Geometry check sheet. Reference: the model listing, model coordinates, mm. A direction names the side the tool comes from. Round coordinates to 2 decimals unless told otherwise and drop trailing zeros. Write each loop counter-clockwise with the first axis right and the second up, starting at its lowest first coordinate (ties: lowest second). Pieces come first, ordered by that corner, then holes. Notation, with made-up numbers: (31, 6.5) -> (78, 6.5) arc R34 ccw to (78, 45.5) -> close; hole circle Ø8 at (-3, 52). An arc over 180 degrees is marked (long way). Return JSON: item names as keys, results as strings. Group by question number.
from build123d import *

# Parameters (mm, degrees)
SKETCH1_W           = 19.05
SKETCH1_H           = 19.05
BOSS_EXTRUDE1_DEPTH = 5.08
SKETCH2_R           = 8.255
BOSS_EXTRUDE2_DEPTH = 15.24
SKETCH3_R           = 6.35
CUT_EXTRUDE1_DEPTH  = 25.379369352
FILLET1_R           = 2.54


with BuildPart() as part:
    # Sketch1 → Boss-Extrude1 (new body)
    with BuildSketch(Plane.XY):
        Rectangle(SKETCH1_W, SKETCH1_H)
    extrude(amount=-BOSS_EXTRUDE1_DEPTH)

    # Sketch2 → Boss-Extrude2 (add)
    with BuildSketch(Plane(origin=(0, 0, -5.08), x_dir=(-1, 0, 0), z_dir=(0, 0, -1))):
        with Locations(Location((0, 0, 0), (0, 0, 180))):
            Circle(SKETCH2_R)
    extrude(amount=BOSS_EXTRUDE2_DEPTH)

    # Sketch3 → Cut-Extrude1 (cut, through all)
    with BuildSketch(Plane.XY):
        Circle(SKETCH3_R)
    extrude(amount=-CUT_EXTRUDE1_DEPTH, mode=Mode.SUBTRACT)

    # Fillet1
    fillet1_edges = [part.edges().sort_by_distance(p)[0] for p in [
        (9.525, -9.525, -2.54),
        (-9.525, -9.525, -2.54),
        (-9.525, 9.525, -2.54),
        (9.525, 9.525, -2.54),
    ]]
    fillet(fillet1_edges, radius=FILLET1_R)


solid = part.part
1) Material ranges on probe 1 along Y at (x, z) = (0, -12.75) (3 decimals); probe 2 along X at (y, z) = (-0.25, -5) (3 decimals); probe 3 along Z at (x, y) = (-4.75, -8.5), recorded low to high. Write a range as [from, to].
2) Mould release check, pull along X, two halves, no side actions. Record for faces 1 (the face through (-8.8, -8.76, -2.58)), 2 (the face through (9.525, 0, -3)), 3 (the face through (-1.38, -6.2, -10.02)), 4 (the face through (0, -9.525, -3)): +X half, -X half, draft (parallel to the pull), parting line (faces both ways), or undercut.
3) Tool access check on faces 5 (the face through (0, 9.525, -3)), 6 (the face through (7.874, -2.48, -12.593)). Record the directions out of +Z, -Z, +X, -X, +Y, -Y that give a thin tool (end or side, any length) a straight path to the whole face; none if there is none.
4) Sectioned sample at C-C on z = -2.75. Enter the section's corners in (x, y) (3 decimals).
5) Sectioned sample at A-A on y = 0. Enter the section's corners in (x, z) (3 decimals), and give its area (3 significant figures).
6) Sectioned sample at D-D on y = 7.75. Enter the section's corners in (x, z), and give its area (3 significant figures).
7) Go/stop test with flat-tipped pins: P1, Ø5, axis at y = -6, z = -9, coming from the +X side; P2, Ø7.5, axis at x = 0, y = 0, coming from the +Z side; P3, Ø8, axis at x = 0.5, z = -14, coming from the -Y side (3 decimals); P4, Ø1, axis at x = 1, z = -13.5, coming from the -Y side. Record where each tip stops, or that it passes through.
Evaluation:
{
 "1": {"probe 1": "y = [-8.255, -6.35], [6.35, 8.255]", "probe 2": "x = [-9.525, -6.345], [6.345, 9.525]", "probe 3": "z = [-5.08, 0]"},
 "2": {"face 1": "-X half", "face 2": "+X half", "face 3": "undercut", "face 4": "draft"},
 "3": {"face 5": "+Z, -Z, +X, -X, +Y", "face 6": "-Z"},
 "4": {"outline": "(-9.525, -6.985) arc R2.54 ccw to (-6.985, -9.525) -> (6.985, -9.525) arc R2.54 ccw to (9.525, -6.985) -> (9.525, 6.985) arc R2.54 ccw to (6.985, 9.525) -> (-6.985, 9.525) arc R2.54 ccw to (-9.525, 6.985) -> close; hole circle Ø12.7 at (0, 0)"},
 "5": {"outline": "(-9.525, -5.08) -> (-8.255, -5.08) -> (-8.255, -20.32) -> (-6.35, -20.32) -> (-6.35, 0) -> (-9.525, 0) -> close; (6.35, -20.32) -> (8.255, -20.32) -> (8.255, -5.08) -> (9.525, -5.08) -> (9.525, 0) -> (6.35, 0) -> close", "area": "90.3 mm2"},
 "6": {"outline": "(-9.41, -5.08) -> (-2.84, -5.08) -> (-2.84, -20.32) -> (2.84, -20.32) -> (2.84, -5.08) -> (9.41, -5.08) -> (9.41, 0) -> (-9.41, 0) -> close", "area": "182 mm2"},
 "7": {"P1": "stops at x = 7.48", "P2": "passes through", "P3": "stops at y = -8.255", "P4": "stops at y = -8.24"}
}
